The listing builds one solid part. Answer for the finished solid, in the listing's coordinates (mm). Face numbers are marked on the shaded views. A direction names the side the tool comes from. Give positions to 0.01 mm unless a question says otherwise; leave off trailing zeros. Use a Markdown table: item, result. Add a question column.
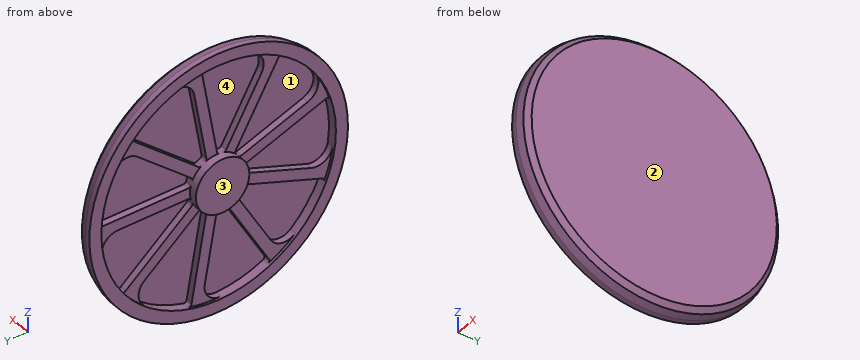
from build123d import *

# Parameters (mm, degrees)
EXTRUDE_1_DEPTH                  = 25
FILLET_3_R                       = 60
FILLET_4_R                       = 10
PATTERN_CIRCULAR_1_COUNT         = 9
FILLET_3_OF_PATTERN_CIRCULAR_1_R = 60
FILLET_4_OF_PATTERN_CIRCULAR_1_R = 10


with BuildPart() as part:
    # 草图1 → 旋转1 (revolve)
    with BuildSketch(Plane.XY, mode=Mode.PRIVATE) as revolve_1_sk:
        Polygon((0, 0), (0, 458.75), (-17.679491924, 476.429491924), (-45, 483.75), (-65, 483.75), (-65, 438.75), (-30, 438.75), (-30, 100), (-85, 100), (-85, 0), align=None)
    revolve(revolve_1_sk.sketch.rotate(Axis((-619.297947583, 0, 0), (1, 0, 0)), 90), axis=Axis((-619.297947583, 0, 0), (1, 0, 0)))

    # 草图3 → 凸台-拉伸1 (add)
    with BuildSketch(Plane.ZY.offset(30)):
        with BuildLine():
            ThreePointArc((20, 438.2939225), (0, 438.75), (-20, 438.2939225))
            Line((-20, 438.2939225), (-20, 97.979589711))
            ThreePointArc((-20, 97.979589711), (0, 100), (20, 97.979589711))
            Line((20, 97.979589711), (20, 438.2939225))
        make_face()
    extrude_1 = extrude(amount=EXTRUDE_1_DEPTH)

    # 圆角3
    fillet_3_edges = [part.edges().sort_by_distance(p)[0] for p in [
        (-42.5, 438.2939225, -20),
    ]]
    fillet(fillet_3_edges, radius=FILLET_3_R)

    # 圆角4
    fillet_4_edges = [part.edges().sort_by_distance(p)[0] for p in [
        (-42.5, 438.2939225, 20),
        (-42.5, 97.979589711, 20),
        (-42.5, 97.979589711, -20),
    ]]
    fillet(fillet_4_edges, radius=FILLET_4_R)

    # 阵列(圆周)1: 凸台-拉伸1 ×9 about axis
    pattern_circular_1_axis = Axis((0, 0, 0), (1, 0, 0))
    for i in range(1, PATTERN_CIRCULAR_1_COUNT):
        add(extrude_1.rotate(pattern_circular_1_axis, i * 360 / PATTERN_CIRCULAR_1_COUNT))

    # 圆角3 of 阵列(圆周)1
    fillet_3_of_pattern_circular_1_edges = [part.edges().sort_by_distance(p)[0] for p in [
        (-42.5, 348.608375977, 266.409013921),
        (-42.5, 95.805095985, 428.162289422),
        (-42.5, -201.826453174, 389.573671209),
        (-42.5, -405.021161842, 168.699202608),
        (-42.5, -418.701967575, -131.111497776),
        (-42.5, -236.467469325, -369.573671209),
        (-42.5, 56.412785864, -435.108216529),
        (-42.5, 322.89687159, -297.050791646),
    ]]
    fillet(fillet_3_of_pattern_circular_1_edges, radius=FILLET_3_OF_PATTERN_CIRCULAR_1_R)

    # 圆角4 of 阵列(圆周)1
    fillet_4_of_pattern_circular_1_edges = [part.edges().sort_by_distance(p)[0] for p in [
        (-42.5, 322.89687159, 297.050791646),
        (-42.5, 62.200968044, 78.300955131),
        (-42.5, 87.912472431, 47.659177406),
        (-42.5, 56.412785864, 435.108216529),
        (-42.5, -2.682177858, 99.964023138),
        (-42.5, 36.710132262, 93.018096031),
        (-42.5, -236.467469325, 369.573671209),
        (-42.5, -66.310302931, 74.852813742),
        (-42.5, -31.66928678, 94.852813742),
        (-42.5, -418.701967575, 131.111497776),
        (-42.5, -98.911100306, 14.7171409),
        (-42.5, -85.230294573, 52.304845732),
        (-42.5, -405.021161842, -168.699202608),
        (-42.5, -85.230294573, -52.304845732),
        (-42.5, -98.911100306, -14.7171409),
        (-42.5, -201.826453174, -389.573671209),
        (-42.5, -31.66928678, -94.852813742),
        (-42.5, -66.310302931, -74.852813742),
        (-42.5, 95.805095985, -428.162289422),
        (-42.5, 36.710132262, -93.018096031),
        (-42.5, -2.682177858, -99.964023138),
        (-42.5, 348.608375977, -266.409013921),
        (-42.5, 87.912472431, -47.659177406),
        (-42.5, 62.200968044, -78.300955131),
    ]]
    fillet(fillet_4_of_pattern_circular_1_edges, radius=FILLET_4_OF_PATTERN_CIRCULAR_1_R)


solid = part.part
1. For a pull along Y with two mould halves and no side action, classify the marked faces 1 and 2 as released by +Y, released by -Y, zero draft, split by the parting line, or undercut.
2. Given P1, Ø5, axis at x = -10.5, y = 57, coming from the +Z side; P2, Ø10, axis at y = 94.5, z = 152, coming from the -X side; P3, Ø8, axis at x = -32.5, y = 179, coming from the +Z side; P4, Ø1.5, axis at y = 178, z = -224.5, coming from the +X side, each flat-ended and moving along its own axis, determine where each tip first touches the part or whether it passes through.
3. Consider L1, parallel to Y at x = -57, z = 0; L2, parallel to Y at x = -51, z = 0; L3, parallel to Y at x = -39, z = 310.5. Determine where each line is inside the solid, lowest interval first. Write a range as [from, to].
4. Which of the six approach directions +Z, -Z, +X, -X, +Y, -Y give full straight-line access (tool end or side, diameter ignored) to the marked faces 3 and 4?
Check values:
| question | item | result |
|---|---|---|
| 1 | face 1 | undercut |
| 1 | face 2 | zero draft |
| 2 | P1 | stops at z = 468.31 |
| 2 | P2 | stops at x = -30 |
| 2 | P3 | stops at z = 447.77 |
| 2 | P4 | stops at x = 0 |
| 3 | L1 | y = [-483.75, -438.75], [-100, 100], [438.75, 483.75] |
| 3 | L2 | y = [-483.75, -438.75], [-100, 483.75] |
| 3 | L3 | y = [-368.85, -309.99], [-202.36, -156.17], [34.44, 75.06], [309.99, 368.85] |
| 4 | face 3 | +Z, -Z, -X, +Y, -Y |
| 4 | face 4 | -X |
